Work out the finished part from the listing and answer in its coordinate system (mm). Face numbers are marked on the shaded views. A direction names the side the tool comes from. Coordinates: 2 decimals unless noted, no trailing zeros. Loops run counter-clockwise (first coordinate to the right, second up) from the corner with the lowest first, then second, coordinate; pieces in that order, holes last. Notation, with made-up numbers: (-34.5, -12) -> (5.5, -12) arc R20 cw to (5.5, 24) -> close; hole circle Ø2 at (74.25, 89). An arc over 180 degrees is marked (long way). Use a Markdown table: item, result.
from build123d import *

# Parameters (mm, degrees)
BOSS_EXTRUDE1_DEPTH = 44.45
SKETCH2_W           = 50.8
SKETCH2_H           = 6.35
BOSS_EXTRUDE2_DEPTH = 68.58
CUT_EXTRUDE1_REACH  = 90.148
SKETCH3_R           = 2.35585
SKETCH4_W           = 101.6
SKETCH4_H           = 9.652
BOSS_EXTRUDE3_DEPTH = 17.78
FILLET1_R           = 10.16


with BuildPart() as part:
    # Sketch1 → Boss-Extrude1 (new body)
    with BuildSketch(Plane.XY):
        Polygon((0, 43.931028897), (50.8, 43.931028897), (50.8, -24.648971103), (57.15, -24.648971103), (57.15, 50.281028897), (0, 50.281028897), align=None)
    boss_extrude1 = extrude(amount=BOSS_EXTRUDE1_DEPTH)

    # Sketch2 → Boss-Extrude2 (add)
    with BuildSketch(Plane.XZ.offset(-43.931028897)):
        with Locations((25.4, 3.175)):
            Rectangle(SKETCH2_W, SKETCH2_H)
    boss_extrude2 = extrude(amount=BOSS_EXTRUDE2_DEPTH)

    # Sketch3 → Cut-Extrude1 (cut, up to next)
    with BuildSketch(Plane(origin=(57.15, 0, 0), x_dir=(0, 0, -1), z_dir=(1, 0, 0)), mode=Mode.PRIVATE) as cut_extrude1_sk1:
        with Locations(Location((-38.608, 24.881028897, 0), (0, 0, 90))):
            Circle(SKETCH3_R)
    cut_extrude1_tool1 = extrude(cut_extrude1_sk1.sketch, amount=-CUT_EXTRUDE1_REACH, mode=Mode.PRIVATE) & part.part
    cut_extrude1 = cut_extrude1_tool1.solids().sort_by_distance((57.15, 24.881029, 38.608))[0]
    add(cut_extrude1, mode=Mode.SUBTRACT)

    # Mirror1: Boss-Extrude1, Boss-Extrude2, Cut-Extrude1 across plane
    add(boss_extrude1.mirror(Plane(origin=(0, 0, 0), x_dir=(0, 0, 1), z_dir=(1, 0, 0))))
    add(boss_extrude2.mirror(Plane(origin=(0, 0, 0), x_dir=(0, 0, 1), z_dir=(1, 0, 0))))
    add(cut_extrude1.mirror(Plane(origin=(0, 0, 0), x_dir=(0, 0, 1), z_dir=(1, 0, 0))), mode=Mode.SUBTRACT)

    # Sketch4 → Boss-Extrude3 (add)
    with BuildSketch(Plane.XY.offset(6.35)):
        with Locations((0, 17.007028897)):
            Rectangle(SKETCH4_W, SKETCH4_H)
    extrude(amount=BOSS_EXTRUDE3_DEPTH)

    # Fillet1
    # the kernel refuses this fillet: 10.16 mm, written as the material it takes off along each edge
    with BuildSketch(Plane(origin=(50.8, 12.181028897, 24.13), x_dir=(0, 1, 0), z_dir=(-1, 0, 0))) as fillet1_piece_1:
        with BuildLine():
            CenterArc((10.16, 10.147292053), FILLET1_R, 180, 87.134016017)
            Line((0, 10.147292053), (0, 0))
            Line((0, 0), (9.652, 0))
        make_face()
    extrude(amount=101.6, mode=Mode.SUBTRACT)


solid = part.part
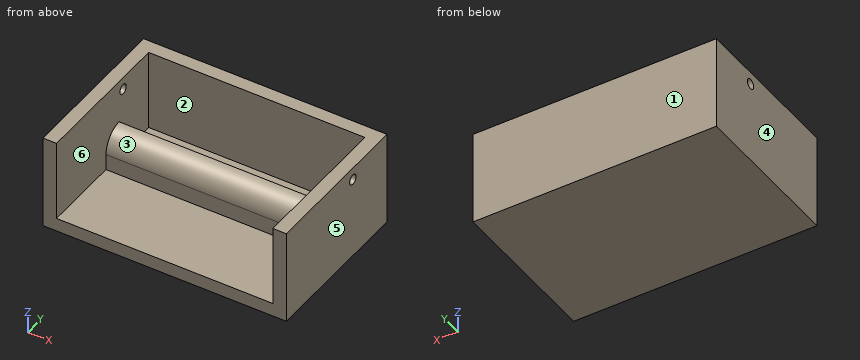
Q1. Consider line 1 (X direction, y = -19.5, z = 30); line 2 (Y direction, x = -39.5, z = 13); line 3 (Z direction, x = 43, y = 41). Determine where each line is inside the solid, lowest interval first. Write a range as [from, to].
Solved:
| item | result |
|---|---|
| line 1 | [-57.15, -50.8], [50.8, 57.15] |
| line 2 | [12.18, 21.83], [43.93, 50.28] |
| line 3 | [0, 6.35] |
Q2. Section C-C on z = 12 is taken. Determine the outline of the cut face in (x, y).
Solved:
| item | result |
|---|---|
| outline | (-57.15, -24.65) -> (-50.8, -24.65) -> (-50.8, 12.18) -> (50.8, 12.18) -> (50.8, -24.65) -> (57.15, -24.65) -> (57.15, 50.28) -> (-57.15, 50.28) -> close; hole (-50.8, 21.83) -> (50.8, 21.83) -> (50.8, 43.93) -> (-50.8, 43.93) -> close |
Q3. Section D-D on z = 30 is taken. Determine the outline of the cut face in (x, y), and give its area (3 significant figures).
Solved:
| item | result |
|---|---|
| outline | (-57.15, -24.65) -> (-50.8, -24.65) -> (-50.8, 43.93) -> (50.8, 43.93) -> (50.8, -24.65) -> (57.15, -24.65) -> (57.15, 50.28) -> (-57.15, 50.28) -> close |
| area | 1,600 mm² |
Q4. Given pin 1 Ø4 at (y, z) = (24.88, 38.61) entering from -X; pin 2 Ø3 at (x, y) = (-27.5, -1) entering from +Z; pin 3 Ø12 at (x, z) = (22, 11.5) entering from -Y; pin 4 Ø2 at (x, y) = (21, 15) entering from +Z, each flat-ended and moving along its own axis, determine where each tip first touches the part or whether it passes through.
Solved:
| item | result |
|---|---|
| pin 1 | through |
| pin 2 | z = 6.35 |
| pin 3 | y = -24.65 |
| pin 4 | z = 21.92 |
Q5. For the marked faces 1, 2 and 3, determine the directions among +Z, -Z, +X, -X, +Y, -Y from which every point of the face is accessible in a straight line to the end or side of a thin tool.
Solved:
| item | result |
|---|---|
| face 1 | +Z, -Z, +X, -X, +Y |
| face 2 | +Z |
| face 3 | +Z, -Y |
Q6. Section A-A on x = 32.5 is taken. Determine the outline of the cut face in (y, z).
Solved:
| item | result |
|---|---|
| outline | (-24.65, 0) -> (50.28, 0) -> (50.28, 44.45) -> (43.93, 44.45) -> (43.93, 6.35) -> (21.83, 6.35) -> (21.83, 24.13) arc R10.16 ccw to (12.18, 13.98) -> (12.18, 6.35) -> (-24.65, 6.35) -> close |
Q7. Determine the mould class of the marked faces 4, 5 and 6 for opening direction X: pulls with the +X half, pulls with the -X half, needs draft (parallel to the pull), parting line crosses it, or undercut.
Solved:
| item | result |
|---|---|
| face 4 | pulls with the -X half |
| face 5 | pulls with the +X half |
| face 6 | undercut |
Q8. Section B-B on y = 6 is taken. Determine the outline of the cut face in (x, z), and give its area (3 significant figures).
Solved:
| item | result |
|---|---|
| outline | (-57.15, 0) -> (57.15, 0) -> (57.15, 44.45) -> (50.8, 44.45) -> (50.8, 6.35) -> (-50.8, 6.35) -> (-50.8, 44.45) -> (-57.15, 44.45) -> close |
| area | 1,210 mm² |
